```python
from build123d import *

# Parameters (mm, degrees)
BOSS_EXTRUDE1_DEPTH = 1.524


with BuildPart() as part:
    # Sketch1 → Boss-Extrude1 (new body)
    with BuildSketch(Plane.XY):
        with BuildLine():
            Line((108.324157749, 0), (107.562157749, 0))
            Line((107.562157749, 0), (106.800157749, 0))
            Line((106.800157749, 0), (106.800157749, -1.524))
            Line((106.800157749, -1.524), (105.512237426, -1.608526345))
            ThreePointArc((105.512237426, -1.608526345), (104.724998688, -3.987284572), (102.691709144, -5.451514459))
            ThreePointArc((102.691709144, -5.451514459), (101.601320714, -5.553518588), (100.569337767, -5.186963043))
            ThreePointArc((100.569337767, -5.186963043), (96.93524901, -1.312980348), (95.693576873, 3.851571261))
            Line((95.693576873, 3.851571261), (95.294914698, 4.01890801))
            Line((95.294914698, 4.01890801), (95.88475327, 5.424136269))
            Line((95.88475327, 5.424136269), (94.479525012, 6.013974841))
            Line((94.479525012, 6.013974841), (93.889686439, 4.608746583))
            Line((93.889686439, 4.608746583), (93.491024264, 4.776083332))
            ThreePointArc((93.491024264, 4.776083332), (93.831172669, 2.518689403), (94.536866699, 0.347624174))
            Line((94.536866699, 0.347624174), (95.57577022, 0.782745178))
            Line((95.57577022, 0.782745178), (95.966908102, -0.770781875))
            Line((95.966908102, -0.770781875), (95.203689029, -1.026803893))
            ThreePointArc((95.203689029, -1.026803893), (98.254836233, -4.783797634), (102.410778326, -7.264250525))
            Line((102.410778326, -7.264250525), (103.161744097, -6.043467632))
            Line((103.161744097, -6.043467632), (104.468983276, -6.847617069))
            Line((104.468983276, -6.847617069), (103.919709272, -7.740526353))
            ThreePointArc((103.919709272, -7.740526353), (104.711489507, -7.917129066), (105.512237426, -8.047156867))
            ThreePointArc((105.512237426, -8.047156867), (107.562157749, -9.102849891), (109.612078072, -8.047156867))
            ThreePointArc((109.612078072, -8.047156867), (110.412825991, -7.917129066), (111.204606226, -7.740526353))
            Line((111.204606226, -7.740526353), (110.655332222, -6.847617069))
            Line((110.655332222, -6.847617069), (111.962571401, -6.043467632))
            Line((111.962571401, -6.043467632), (112.713537171, -7.264250525))
            ThreePointArc((112.713537171, -7.264250525), (116.869479265, -4.783797634), (119.920626468, -1.026803893))
            Line((119.920626468, -1.026803893), (119.157407395, -0.770781875))
            Line((119.157407395, -0.770781875), (119.548545278, 0.782745178))
            Line((119.548545278, 0.782745178), (120.587448799, 0.347624174))
            ThreePointArc((120.587448799, 0.347624174), (121.293142829, 2.518689403), (121.633291234, 4.776083332))
            Line((121.633291234, 4.776083332), (121.234629058, 4.608746583))
            Line((121.234629058, 4.608746583), (120.644790486, 6.013974841))
            Line((120.644790486, 6.013974841), (119.239562227, 5.424136269))
            Line((119.239562227, 5.424136269), (119.8294008, 4.01890801))
            Line((119.8294008, 4.01890801), (119.430738625, 3.851571261))
            ThreePointArc((119.430738625, 3.851571261), (118.189066488, -1.312980348), (114.55497773, -5.186963043))
            ThreePointArc((114.55497773, -5.186963043), (113.522994784, -5.553518588), (112.432606354, -5.451514459))
            ThreePointArc((112.432606354, -5.451514459), (110.399316809, -3.987284572), (109.612078072, -1.608526345))
            Line((109.612078072, -1.608526345), (108.324157749, -1.524))
            Line((108.324157749, -1.524), (108.324157749, 0))
        make_face()
    extrude(amount=BOSS_EXTRUDE1_DEPTH)


solid = part.part
```
Work out the finished part from the listing and answer in its coordinate system (mm). A direction names the side the tool comes from. Give positions to 0.01 mm unless a question says otherwise; leave off trailing zeros. Loops run counter-clockwise (first coordinate to the right, second up) from the corner with the lowest first, then second, coordinate; pieces in that order, holes last. Notation, with made-up numbers: (30.5, -5.5) -> (66.5, -5.5) arc R11 cw to (66.5, -0.5) -> close; hole circle Ø5 at (-16, 89). An arc over 180 degrees is marked (long way). Write item = value, one per line. Start each with the question number.
(1) Which of the six approach directions +Z, -Z, +X, -X, +Y, -Y give full straight-line access (tool end or side, diameter ignored) to faces 1 (the flat face through (102.781, -6.662, 0.751)), 2 (the flat face through (108.977, -1.567, 0.751)), 3 (the cylindrical face through (121.286, 2.488, 0.751)), 4 (the flat face through (119.35, 0, 0.75))?
(2) Find section C-C on x = 108. Give the vertices of the cut face in (y, z).
(3) Given pin 1 Ø0.5 at (y, z) = (-0.5, 0.5) entering from -X, flat-ended and moving along its own axis, determine where the tip first touches the part or whether it passes through.
(4) The mould has two halves that part along Y. Classify faces 5 (the cylindrical face through (98.203, -4.739, 0.751)), 6 (the flat face through (108, 0, 1)), 7 (the flat face through (95.049, 0.562, 0.751)): +Y half, -Y half, draft (parallel to the pull), parting line (faces both ways), or undercut.
(5) Find section D-D on x = 116.5. Give the vertices of the cut face in (y, z).
(6) Find section B-B on y = -3.25. Give the vertices of the cut face in (x, z), and give its area (3 significant figures).
(7) Find the intervals of material crossed by probe 1 along X at (y, z) = (-7, 1.1); probe 2 along X at (y, z) = (-4, 1.1); probe 3 along X at (y, z) = (0.5, 0.85), in increasing order. Write a range as from..to.
(8) Find section A-A on y = 3.25. Give the vertices of the cut face in (x, z), and give its area (3 significant figures).
From the geometry:
q1.face_1 = +Z, -Z, -Y
q1.face_2 = +Z, -Z, +Y
q1.face_3 = +Z, -Z, +X, -Y
q1.face_4 = +Z, -Z
q2.outline = (-9.06, 0) -> (0, 0) -> (0, 1.52) -> (-9.06, 1.52) -> close
q3.pin_1 = 95.84
q4.face_5 = -Y half
q4.face_6 = +Y half
q4.face_7 = undercut
q5.outline = (-5.09, 0) -> (-3.62, 0) -> (-3.62, 1.52) -> (-5.09, 1.52) -> close
q6.outline = (96.74, 0) -> (98.29, 0) -> (98.29, 1.52) -> (96.74, 1.52) -> close; (105.15, 0) -> (109.97, 0) -> (109.97, 1.52) -> (105.15, 1.52) -> close; (116.84, 0) -> (118.39, 0) -> (118.39, 1.52) -> (116.84, 1.52) -> close
q6.area = 12.1 mm^2
q7.probe_1 = 101.76..102.57, 104.38..110.75, 112.55..113.36
q7.probe_2 = 97.42..99.02, 104.72..110.41, 116.11..117.7
q7.probe_3 = 94.47..94.9, 95.65..96.17, 118.96..119.48, 120.22..120.65
q8.outline = (93.68, 0) -> (95.7, 0) -> (95.7, 1.52) -> (93.68, 1.52) -> close; (119.43, 0) -> (121.45, 0) -> (121.45, 1.52) -> (119.43, 1.52) -> close
q8.area = 6.15 mm^2
